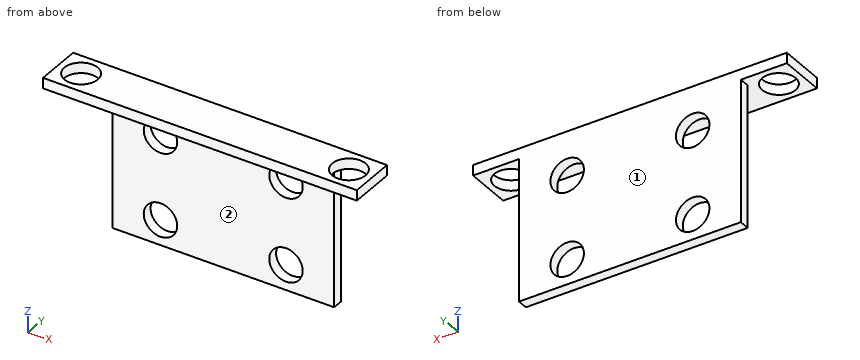
from build123d import *

# Parameters (mm, degrees)
SKETCH_1_W      = 53
SKETCH_1_H      = 36.5
SKETCH_1_R      = 4
EXTRUDE_1_DEPTH = 2.5
SKETCH_2_W      = 75
SKETCH_2_H      = 11
SKETCH_2_R      = 4
EXTRUDE_2_DEPTH = 2.5


with BuildPart() as part:
    # 草图1 → 凸台-拉伸1 (new body)
    with BuildSketch(Plane(origin=(0, 0, 0), x_dir=(1, 0, 0), z_dir=(0, 1, 0))):
        with Locations((13.886189258, -1.177109974)):
            Rectangle(SKETCH_1_W, SKETCH_1_H)
        with Locations(Location((-1.113810742, 11.072890026, 0), (0, 0, 270))):
            Circle(SKETCH_1_R, mode=Mode.SUBTRACT)
        with Locations(Location((28.886189258, 11.072890026, 0), (0, 0, 270))):
            Circle(SKETCH_1_R, mode=Mode.SUBTRACT)
        with Locations(Location((28.886189258, -8.927109974, 0), (0, 0, 270))):
            Circle(SKETCH_1_R, mode=Mode.SUBTRACT)
        with Locations(Location((-1.113810742, -8.927109974, 0), (0, 0, 270))):
            Circle(SKETCH_1_R, mode=Mode.SUBTRACT)
    extrude(amount=EXTRUDE_1_DEPTH)

    # 草图2 → 凸台-拉伸2 (add)
    with BuildSketch(Plane.XY.offset(19.427109974)):
        with Locations((13.886189258, -3)):
            Rectangle(SKETCH_2_W, SKETCH_2_H)
        with Locations((-18.113810742, -3)):
            Circle(SKETCH_2_R, mode=Mode.SUBTRACT)
        with Locations((45.886189258, -3)):
            Circle(SKETCH_2_R, mode=Mode.SUBTRACT)
    extrude(amount=-EXTRUDE_2_DEPTH)


solid = part.part
Part model, mm, in its own coordinate system. Face numbers are marked on the shaded views. A direction names the side the tool comes from. Round coordinates to 2 decimals unless told otherwise and drop trailing zeros. Write each loop counter-clockwise with the first axis right and the second up, starting at its lowest first coordinate (ties: lowest second). Pieces come first, ordered by that corner, then holes. Notation, with made-up numbers: M -26,28 L 5,28 A10 ccw 5,40 Z; hole C -20.75,30 d11. An arc over 180 degrees is marked long. Return JSON: item names as keys, results as strings. Group by question number.
(1) Saw through at A-A on z = 12. Write the cut outline in (x, y), then the cut area to 3 significant figures.
(2) Saw through at C-C on x = 22. Write the cut outline in (y, z), then the cut area to 4 significant figures.
(3) Saw through at B-B on y = -3. Write the cut outline in (x, z).
(4) Drill centre lines: probe 1 along Y at (x, z) = (24.5, 12.5); probe 2 along Z at (x, y) = (30.5, -5.5); probe 3 along X at (y, z) = (2, -7). Where is each one in solid material? Low to high.
(5) Pin check, flat tips, straight feed: pin 1 Ø6.5 at (x, z) = (-1.11, -11.07) entering from +Y; pin 2 Ø5.5 at (x, y) = (11.5, -5.5) entering from -Z; pin 3 Ø3 at (y, z) = (-1, -4.5) entering from +X; pin 4 Ø3 at (y, z) = (1.5, -7.5) entering from -X. Stop position of each tip, or through.
(6) Which spindle directions (+Z, -Z, +X, -X, +Y, -Y) get a long thin tool onto all of the face, cutting with end or side? Do the marked faces 1 and 2. Say none if no direction does.
Returned:
{
 "1": {"outline": "M -12.61,0 L -3.67,0 L -3.67,2.5 L -12.61,2.5 Z; M 1.45,0 L 26.33,0 L 26.33,2.5 L 1.45,2.5 Z; M 31.45,0 L 40.39,0 L 40.39,2.5 L 31.45,2.5 Z", "area": "107 mm²"},
 "2": {"outline": "M -8.5,16.93 L 0,16.93 L 0,-17.07 L 2.5,-17.07 L 2.5,19.43 L -8.5,19.43 Z", "area": "112.5 mm²"},
 "3": {"outline": "M -23.61,16.93 L -22.11,16.93 L -22.11,19.43 L -23.61,19.43 Z; M -14.11,16.93 L 41.89,16.93 L 41.89,19.43 L -14.11,19.43 Z; M 49.89,16.93 L 51.39,16.93 L 51.39,19.43 L 49.89,19.43 Z"},
 "4": {"probe 1": "0 to 2.5", "probe 2": "16.93 to 19.43", "probe 3": "-12.61 to 40.39"},
 "5": {"pin 1": "through", "pin 2": "z = 16.93", "pin 3": "x = 40.39", "pin 4": "x = -12.61"},
 "6": {"face 1": "+Z, -Z, +X, -X, +Y", "face 2": "-Z, +X, -X, -Y"}
}
